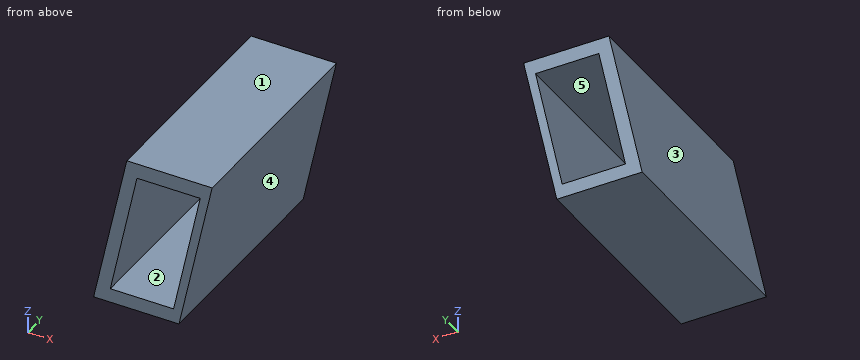
```python
from build123d import *

# Parameters (mm, degrees)
F1_DEPTH = 76.2
F3_DEPTH = 38.1
F4_DEPTH = 38.1


with BuildPart() as f1:
    # F0 (on Front) → F1 (new body)
    with BuildSketch(Plane.XZ):
        Polygon((13.32986, 63.908778), (-16.15954, 63.908778), (-27.629351, 10.361006), (1.860049, 10.361006), align=None)
    extrude(amount=F1_DEPTH)

    # F2 (on Front) → F3 (cut, symmetric)
    with BuildSketch(Plane.XZ):
        Polygon((9.213624, 58.712374), (-12.659614, 58.712374), (-21.8694, 15.253705), (0, 15.253705), align=None)
    extrude(amount=F3_DEPTH, both=True, mode=Mode.SUBTRACT)

    # F3_face (on face) → F4 (cut, symmetric)
    with BuildSketch(Plane(origin=(-6.328713, -38.1, 36.983675), x_dir=(1, 0, 0), z_dir=(0, 1, 0))):
        Polygon((15.542337, -21.728699), (6.328713, 21.72997), (-15.540687, 21.72997), (-6.330902, -21.728699), align=None)
    extrude(amount=F4_DEPTH, both=True, mode=Mode.SUBTRACT)


solid = f1.part
```
Input: part model. Units: mm. Frame: model coordinates. Face numbers are marked on the shaded views. A direction names the side the tool comes from. Give positions to 0.01 mm unless a question says otherwise; leave off trailing zeros. Order: outer loops, then holes, each group sorted by start corner. A loop starts at its lowest first (then second) coordinate and runs counter-clockwise, first axis right, second up. Notation, with made-up numbers: M 57.5,22 L 111.5,22 A38 ccw 111.5,61 Z; hole C 60,18 d11. An arc over 180 degrees is marked long. Return JSON: item names as keys, results as strings.
1) Section query A-A on x = -11. Output: boundary loops of the cut face in (y, z).
Taken from the geometry:
{"outline": "M -76.2,10.36 L 0,10.36 L 0,15.25 L -76.2,15.25 Z; M -76.2,58.71 L 0,58.71 L 0,63.91 L -76.2,63.91 Z"}
2) Contact query for flat-ended pins moving along their axis: pin 1 (12 mm diameter, centred on y = -9, z = 49.5, fed in from +X); pin 2 (12 mm diameter, centred on y = -32.5, z = 46.5, fed in from +X); pin 3 (10 mm diameter, centred on y = -62, z = 46, fed in from +X). Output: stop coordinate, or through.
Taken from the geometry:
{"pin 1": "stops at x = 11.53", "pin 2": "stops at x = 10.89", "pin 3": "stops at x = 10.56"}
3) Section query B-B on z = 31.5. Output: boundary loops of the cut face in (x, y), and give its area (3 significant figures).
Taken from the geometry:
{"outline": "M -23.1,-76.2 L -18.43,-76.2 L -18.43,0 L -23.1,0 Z; M 3.44,-76.2 L 6.39,-76.2 L 6.39,0 L 3.44,0 Z", "area": "581 mm2"}
4) Access query for the marked faces 4 and 5. Directions: +Z, -Z, +X, -X, +Y, -Y. A direction counts if a zero-diameter tool reaches every point of the face in a straight line with its end or side. Return the directions, or none.
Taken from the geometry:
{"face 4": "-Z, +X, +Y, -Y", "face 5": "+Y, -Y"}
5) Line query: L1, parallel to Z at x = -0.5, y = -34.5; L2, parallel to X at y = -28.5, z = 19; L3, parallel to X at y = -53.5, z = 45.5. Output: solid intervals per line, ascending. Write a range as [from, to].
Taken from the geometry:
{"L1": "z = [10.36, 15.25], [58.71, 63.91]", "L2": "x = [-25.78, -21.08], [0.79, 3.71]", "L3": "x = [-20.1, -15.46], [6.41, 9.39]"}
6) Section query C-C on y = -53.5. Output: boundary loops of the cut face in (x, z).
Taken from the geometry:
{"outline": "M -27.63,10.36 L 1.86,10.36 L 13.33,63.91 L -16.16,63.91 Z; hole M -21.87,15.25 L 0,15.25 L 9.21,58.71 L -12.66,58.71 Z"}
7) Mould query, pull axis X, two halves, no side actions, for the marked faces 1, 2 and 3. Classes: released by +X, released by -X, zero draft, split by the parting line, or undercut.
Taken from the geometry:
{"face 1": "zero draft", "face 2": "undercut", "face 3": "released by -X"}
8) Section query D-D on x = -24.5. Output: boundary loops of the cut face in (y, z), and give its area (3 significant figures).
Taken from the geometry:
{"outline": "M -76.2,10.36 L 0,10.36 L 0,24.97 L -76.2,24.97 Z", "area": "1,110 mm2"}
